from build123d import *

# Parameters (mm, degrees)
SKETCH2_R           = 250
SKETCH2_R_2         = 5.1
SKETCH2_R_3         = 75.5
SKETCH2_R_4         = 1.25
SKETCH2_R_5         = 1.6
SKETCH2_R_6         = 2
BOSS_EXTRUDE1_DEPTH = 2.5


with BuildPart() as part:
    # Sketch2 → Boss-Extrude1 (new, symmetric)
    with BuildSketch(Plane(origin=(0, 0, 0), x_dir=(1, 0, 0), z_dir=(0, 1, 0))):
        with Locations(Location((0, 0, 0), (0, 0, 270))):
            Circle(SKETCH2_R)
        with Locations(Location((0, 222.5, 0), (0, 0, 270))):
            Circle(SKETCH2_R_2, mode=Mode.SUBTRACT)
        with Locations(Location((0, 0, 0), (0, 0, 270))):
            Circle(SKETCH2_R_3, mode=Mode.SUBTRACT)
        with Locations(Location((4, 79.899937422, 0), (0, 0, 270))):
            Circle(SKETCH2_R_4, mode=Mode.SUBTRACT)
        with Locations(Location((-4, 79.899937422, 0), (0, 0, 90))):
            Circle(SKETCH2_R_4, mode=Mode.SUBTRACT)
        with Locations(Location((16.815922202, 78.212689255, 0), (0, 0, 90))):
            Circle(SKETCH2_R_4, mode=Mode.SUBTRACT)
        with Locations(Location((24.543328812, 76.142136894, 0), (0, 0, 270))):
            Circle(SKETCH2_R_4, mode=Mode.SUBTRACT)
        with Locations(Location((36.485867096, 71.195375568, 0), (0, 0, 90))):
            Circle(SKETCH2_R_4, mode=Mode.SUBTRACT)
        with Locations(Location((43.414070326, 67.195375568, 0), (0, 0, 270))):
            Circle(SKETCH2_R_4, mode=Mode.SUBTRACT)
        with Locations(Location((53.669360443, 59.326214692, 0), (0, 0, 90))):
            Circle(SKETCH2_R_4, mode=Mode.SUBTRACT)
        with Locations(Location((59.326214692, 53.669360443, 0), (0, 0, 270))):
            Circle(SKETCH2_R_4, mode=Mode.SUBTRACT)
        with Locations(Location((67.195375568, 43.414070326, 0), (0, 0, 90))):
            Circle(SKETCH2_R_4, mode=Mode.SUBTRACT)
        with Locations(Location((71.195375568, 36.485867096, 0), (0, 0, 270))):
            Circle(SKETCH2_R_4, mode=Mode.SUBTRACT)
        with Locations(Location((76.142136894, 24.543328812, 0), (0, 0, 90))):
            Circle(SKETCH2_R_4, mode=Mode.SUBTRACT)
        with Locations(Location((78.212689255, 16.815922202, 0), (0, 0, 270))):
            Circle(SKETCH2_R_4, mode=Mode.SUBTRACT)
        with Locations(Location((79.899937422, 4, 0), (0, 0, 90))):
            Circle(SKETCH2_R_4, mode=Mode.SUBTRACT)
        with Locations(Location((79.899937422, -4, 0), (0, 0, 270))):
            Circle(SKETCH2_R_4, mode=Mode.SUBTRACT)
        with Locations(Location((78.212689255, -16.815922202, 0), (0, 0, 90))):
            Circle(SKETCH2_R_4, mode=Mode.SUBTRACT)
        with Locations(Location((76.142136894, -24.543328812, 0), (0, 0, 270))):
            Circle(SKETCH2_R_4, mode=Mode.SUBTRACT)
        with Locations(Location((192.690652342, 111.25, 0), (0, 0, 270))):
            Circle(SKETCH2_R_2, mode=Mode.SUBTRACT)
        with Locations(Location((192.690652342, -111.25, 0), (0, 0, 270))):
            Circle(SKETCH2_R_2, mode=Mode.SUBTRACT)
        with Locations(Location((0, -222.5, 0), (0, 0, 270))):
            Circle(SKETCH2_R_2, mode=Mode.SUBTRACT)
        with Locations(Location((-192.690652342, -111.25, 0), (0, 0, 270))):
            Circle(SKETCH2_R_2, mode=Mode.SUBTRACT)
        with Locations(Location((-192.690652342, 111.25, 0), (0, 0, 270))):
            Circle(SKETCH2_R_2, mode=Mode.SUBTRACT)
        with Locations(Location((-41.042417199, 112.763114494, 0), (0, 0, 270))):
            Circle(SKETCH2_R_5, mode=Mode.SUBTRACT)
        with Locations(Location((-34.202014333, 93.969262079, 0), (0, 0, 270))):
            Circle(SKETCH2_R_5, mode=Mode.SUBTRACT)
        with Locations(Location((41.042417199, 112.763114494, 0), (0, 0, 90))):
            Circle(SKETCH2_R_5, mode=Mode.SUBTRACT)
        with Locations(Location((34.202014333, 93.969262079, 0), (0, 0, 90))):
            Circle(SKETCH2_R_5, mode=Mode.SUBTRACT)
        with Locations(Location((90.630778704, 42.261826174, 0), (0, 0, 90))):
            Circle(SKETCH2_R_5, mode=Mode.SUBTRACT)
        with Locations(Location((42.261826174, 90.630778704, 0), (0, 0, 270))):
            Circle(SKETCH2_R_5, mode=Mode.SUBTRACT)
        with Locations(Location((50.714191409, 108.756934444, 0), (0, 0, 270))):
            Circle(SKETCH2_R_5, mode=Mode.SUBTRACT)
        with Locations(Location((108.756934444, 50.714191409, 0), (0, 0, 90))):
            Circle(SKETCH2_R_5, mode=Mode.SUBTRACT)
        with Locations(Location((93.969262079, -34.202014333, 0), (0, 0, 90))):
            Circle(SKETCH2_R_5, mode=Mode.SUBTRACT)
        with Locations(Location((93.969262079, 34.202014333, 0), (0, 0, 270))):
            Circle(SKETCH2_R_5, mode=Mode.SUBTRACT)
        with Locations(Location((112.763114494, 41.042417199, 0), (0, 0, 270))):
            Circle(SKETCH2_R_5, mode=Mode.SUBTRACT)
        with Locations(Location((112.763114494, -41.042417199, 0), (0, 0, 90))):
            Circle(SKETCH2_R_5, mode=Mode.SUBTRACT)
        with Locations(Location((42.261826174, -90.630778704, 0), (0, 0, 90))):
            Circle(SKETCH2_R_5, mode=Mode.SUBTRACT)
        with Locations(Location((90.630778704, -42.261826174, 0), (0, 0, 270))):
            Circle(SKETCH2_R_5, mode=Mode.SUBTRACT)
        with Locations(Location((108.756934444, -50.714191409, 0), (0, 0, 270))):
            Circle(SKETCH2_R_5, mode=Mode.SUBTRACT)
        with Locations(Location((50.714191409, -108.756934444, 0), (0, 0, 90))):
            Circle(SKETCH2_R_5, mode=Mode.SUBTRACT)
        with Locations(Location((-34.202014333, -93.969262079, 0), (0, 0, 90))):
            Circle(SKETCH2_R_5, mode=Mode.SUBTRACT)
        with Locations(Location((34.202014333, -93.969262079, 0), (0, 0, 270))):
            Circle(SKETCH2_R_5, mode=Mode.SUBTRACT)
        with Locations(Location((41.042417199, -112.763114494, 0), (0, 0, 270))):
            Circle(SKETCH2_R_5, mode=Mode.SUBTRACT)
        with Locations(Location((-41.042417199, -112.763114494, 0), (0, 0, 90))):
            Circle(SKETCH2_R_5, mode=Mode.SUBTRACT)
        with Locations(Location((-90.630778704, -42.261826174, 0), (0, 0, 90))):
            Circle(SKETCH2_R_5, mode=Mode.SUBTRACT)
        with Locations(Location((-42.261826174, -90.630778704, 0), (0, 0, 270))):
            Circle(SKETCH2_R_5, mode=Mode.SUBTRACT)
        with Locations(Location((-50.714191409, -108.756934444, 0), (0, 0, 270))):
            Circle(SKETCH2_R_5, mode=Mode.SUBTRACT)
        with Locations(Location((-108.756934444, -50.714191409, 0), (0, 0, 90))):
            Circle(SKETCH2_R_5, mode=Mode.SUBTRACT)
        with Locations(Location((-93.969262079, 34.202014333, 0), (0, 0, 90))):
            Circle(SKETCH2_R_5, mode=Mode.SUBTRACT)
        with Locations(Location((-93.969262079, -34.202014333, 0), (0, 0, 270))):
            Circle(SKETCH2_R_5, mode=Mode.SUBTRACT)
        with Locations(Location((-112.763114494, -41.042417199, 0), (0, 0, 270))):
            Circle(SKETCH2_R_5, mode=Mode.SUBTRACT)
        with Locations(Location((-112.763114494, 41.042417199, 0), (0, 0, 90))):
            Circle(SKETCH2_R_5, mode=Mode.SUBTRACT)
        with Locations(Location((-42.261826174, 90.630778704, 0), (0, 0, 90))):
            Circle(SKETCH2_R_5, mode=Mode.SUBTRACT)
        with Locations(Location((-90.630778704, 42.261826174, 0), (0, 0, 270))):
            Circle(SKETCH2_R_5, mode=Mode.SUBTRACT)
        with Locations(Location((-108.756934444, 50.714191409, 0), (0, 0, 270))):
            Circle(SKETCH2_R_5, mode=Mode.SUBTRACT)
        with Locations(Location((-50.714191409, 108.756934444, 0), (0, 0, 90))):
            Circle(SKETCH2_R_5, mode=Mode.SUBTRACT)
        with Locations(Location((71.195375568, -36.485867096, 0), (0, 0, 90))):
            Circle(SKETCH2_R_4, mode=Mode.SUBTRACT)
        with Locations(Location((67.195375568, -43.414070326, 0), (0, 0, 270))):
            Circle(SKETCH2_R_4, mode=Mode.SUBTRACT)
        with Locations(Location((59.326214692, -53.669360443, 0), (0, 0, 90))):
            Circle(SKETCH2_R_4, mode=Mode.SUBTRACT)
        with Locations(Location((53.669360443, -59.326214692, 0), (0, 0, 270))):
            Circle(SKETCH2_R_4, mode=Mode.SUBTRACT)
        with Locations(Location((43.414070326, -67.195375568, 0), (0, 0, 90))):
            Circle(SKETCH2_R_4, mode=Mode.SUBTRACT)
        with Locations(Location((36.485867096, -71.195375568, 0), (0, 0, 270))):
            Circle(SKETCH2_R_4, mode=Mode.SUBTRACT)
        with Locations(Location((24.543328812, -76.142136894, 0), (0, 0, 90))):
            Circle(SKETCH2_R_4, mode=Mode.SUBTRACT)
        with Locations(Location((16.815922202, -78.212689255, 0), (0, 0, 270))):
            Circle(SKETCH2_R_4, mode=Mode.SUBTRACT)
        with Locations(Location((4, -79.899937422, 0), (0, 0, 90))):
            Circle(SKETCH2_R_4, mode=Mode.SUBTRACT)
        with Locations(Location((-4, -79.899937422, 0), (0, 0, 270))):
            Circle(SKETCH2_R_4, mode=Mode.SUBTRACT)
        with Locations(Location((-16.815922202, -78.212689255, 0), (0, 0, 90))):
            Circle(SKETCH2_R_4, mode=Mode.SUBTRACT)
        with Locations(Location((-24.543328812, -76.142136894, 0), (0, 0, 270))):
            Circle(SKETCH2_R_4, mode=Mode.SUBTRACT)
        with Locations(Location((-36.485867096, -71.195375568, 0), (0, 0, 90))):
            Circle(SKETCH2_R_4, mode=Mode.SUBTRACT)
        with Locations(Location((-43.414070326, -67.195375568, 0), (0, 0, 270))):
            Circle(SKETCH2_R_4, mode=Mode.SUBTRACT)
        with Locations(Location((-53.669360442, -59.326214692, 0), (0, 0, 90))):
            Circle(SKETCH2_R_4, mode=Mode.SUBTRACT)
        with Locations(Location((-59.326214692, -53.669360443, 0), (0, 0, 270))):
            Circle(SKETCH2_R_4, mode=Mode.SUBTRACT)
        with Locations(Location((-67.195375568, -43.414070326, 0), (0, 0, 90))):
            Circle(SKETCH2_R_4, mode=Mode.SUBTRACT)
        with Locations(Location((-71.195375568, -36.485867096, 0), (0, 0, 270))):
            Circle(SKETCH2_R_4, mode=Mode.SUBTRACT)
        with Locations(Location((-76.142136894, -24.543328812, 0), (0, 0, 90))):
            Circle(SKETCH2_R_4, mode=Mode.SUBTRACT)
        with Locations(Location((-78.212689255, -16.815922202, 0), (0, 0, 270))):
            Circle(SKETCH2_R_4, mode=Mode.SUBTRACT)
        with Locations(Location((-79.899937422, -4, 0), (0, 0, 90))):
            Circle(SKETCH2_R_4, mode=Mode.SUBTRACT)
        with Locations(Location((-79.899937422, 4, 0), (0, 0, 270))):
            Circle(SKETCH2_R_4, mode=Mode.SUBTRACT)
        with Locations(Location((-78.212689255, 16.815922202, 0), (0, 0, 90))):
            Circle(SKETCH2_R_4, mode=Mode.SUBTRACT)
        with Locations(Location((-76.142136894, 24.543328812, 0), (0, 0, 270))):
            Circle(SKETCH2_R_4, mode=Mode.SUBTRACT)
        with Locations(Location((-71.195375568, 36.485867096, 0), (0, 0, 90))):
            Circle(SKETCH2_R_4, mode=Mode.SUBTRACT)
        with Locations(Location((-67.195375568, 43.414070326, 0), (0, 0, 270))):
            Circle(SKETCH2_R_4, mode=Mode.SUBTRACT)
        with Locations(Location((-59.326214692, 53.669360443, 0), (0, 0, 90))):
            Circle(SKETCH2_R_4, mode=Mode.SUBTRACT)
        with Locations(Location((-53.669360443, 59.326214692, 0), (0, 0, 270))):
            Circle(SKETCH2_R_4, mode=Mode.SUBTRACT)
        with Locations(Location((-43.414070326, 67.195375568, 0), (0, 0, 90))):
            Circle(SKETCH2_R_4, mode=Mode.SUBTRACT)
        with Locations(Location((-36.485867096, 71.195375568, 0), (0, 0, 270))):
            Circle(SKETCH2_R_4, mode=Mode.SUBTRACT)
        with Locations(Location((-24.543328812, 76.142136894, 0), (0, 0, 90))):
            Circle(SKETCH2_R_4, mode=Mode.SUBTRACT)
        with Locations(Location((-16.815922202, 78.212689255, 0), (0, 0, 270))):
            Circle(SKETCH2_R_4, mode=Mode.SUBTRACT)
        with Locations(Location((-129.383554409, -17.033668085, 0), (0, 0, 270))):
            Circle(SKETCH2_R_6, mode=Mode.SUBTRACT)
        with Locations(Location((-130.5, 0, 0), (0, 0, 270))):
            Circle(SKETCH2_R_6, mode=Mode.SUBTRACT)
        with Locations(Location((129.383554409, 17.033668085, 0), (0, 0, 90))):
            Circle(SKETCH2_R_6, mode=Mode.SUBTRACT)
        with Locations(Location((126.053320331, 33.775885386, 0), (0, 0, 90))):
            Circle(SKETCH2_R_6, mode=Mode.SUBTRACT)
    extrude(amount=BOSS_EXTRUDE1_DEPTH, both=True)


solid = part.part
Read the model definition and answer for the solid it produces. Units are mm, in the model's axes. Give positions to 0.01 mm unless a question says otherwise; leave off trailing zeros. Loops run counter-clockwise (first coordinate to the right, second up) from the corner with the lowest first, then second, coordinate; pieces in that order, holes last. Notation, with made-up numbers: M -17,-13 L 39,-13 A19 cw 39,16 Z; hole C 87.25,80 d5. An arc over 180 degrees is marked long. Write each question's results on one line, items separated by ' | '.
1. Section A-A on y = -0.6 is taken. State how many separate pieces and enclosed holes the cut face has, plus the area to 3 significant figures.
Values:
separate pieces: 1 | enclosed holes: 91 | area: 177,000 mm^2
2. The mould has two halves that part along Z. Classify faces 1 (the face through (22.678, -0.035, 72.014)), 2 (the face through (59, -2.5, 52)), 3 (the face through (10.99, 0.04, -249.76)): pulls with the +Z half, pulls with the -Z half, needs draft (parallel to the pull), parting line crosses it, or undercut.
Values:
face 1: undercut | face 2: needs draft | face 3: parting line crosses it
3. Given pin 1 (3 mm diameter, centred on x = -76.14, z = -24.54, fed in from -Y); pin 2 (2 mm diameter, centred on x = 43.41, z = 67.2, fed in from +Y); pin 3 (3 mm diameter, centred on y = -1, z = 127, fed in from -X); pin 4 (2 mm diameter, centred on x = 79, y = -1, fed in from -Z), each flat-ended and moving along its own axis, determine where each tip first touches the part or whether it passes through.
Values:
pin 1: stops at y = -2.5 | pin 2: passes through | pin 3: stops at x = -216.22 | pin 4: stops at z = -237.52
4. Section B-B on x = -154.5 is taken. Give the vertices of the cut face in (y, z).
Values:
outline: M -2.5,-196.54 L 2.5,-196.54 L 2.5,196.54 L -2.5,196.54 Z
5. Section C-C on z = -185.5 is taken. Give the vertices of the cut face in (x, y), plus the area to 3 significant figures.
Values:
outline: M -167.6,-2.5 L 167.6,-2.5 L 167.6,2.5 L -167.6,2.5 Z | area: 1,680 mm^2
6. Straight lines are drawn through the part: line 1 (X direction, y = -1.1, z = 4); line 2 (X direction, y = -1.55, z = -0.5); line 3 (X direction, y = 1.7, z = -34.5). For each, find the intervals that lie inside material, in ascending order. Write a range as [from, to].
Values:
line 1: x = [-249.97, -81.15], [-78.65, -75.39], [75.39, 78.65], [81.15, 249.97] | line 2: x = [-250, -132.44], [-128.56, -75.5], [75.5, 250] | line 3: x = [-247.61, -95.54], [-92.4, -67.16], [67.16, 92.4], [95.54, 124.19], [127.92, 247.61]
